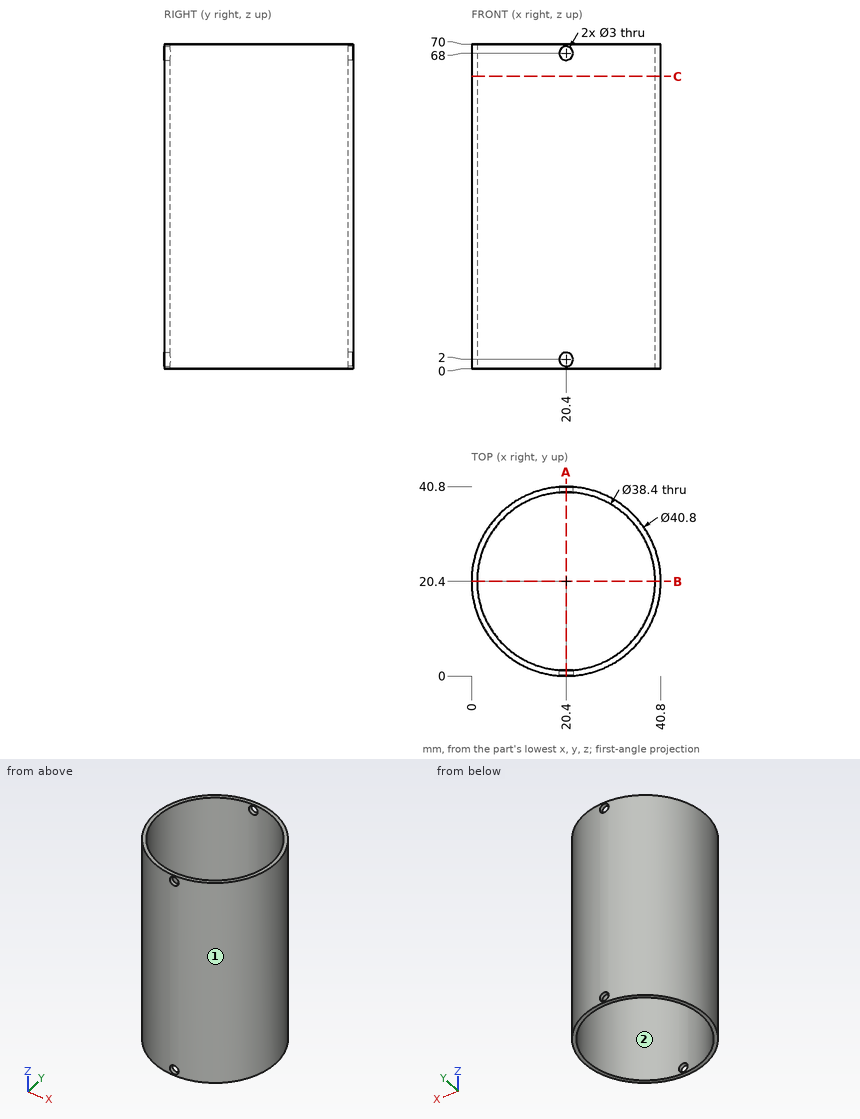
Design review of the part shown in the three views and the two pictorial views. Dimensions are in mm from the part's minimum x, y and z. Give positions to 0.01 mm unless a question says otherwise; leave off trailing zeros. Loops run counter-clockwise (first coordinate to the right, second up) from the corner with the lowest first, then second, coordinate; pieces in that order, holes last. Notation, with made-up numbers: (36.25, 88.25) -> (45.25, 88.25) arc R22 cw to (45.25, 108.25) -> close; hole circle Ø1 at (41.5, 32.5). An arc over 180 degrees is marked (long way). One line per item, written item: value.
Q1. We need section C-C on z = 63. Give the boundary of the cut face in (x, y).
Numbers:
outline: circle Ø40.8 at (20.4, 20.4); hole circle Ø38.4 at (20.4, 20.4)
Q2. We need section A-A on x = 20.4. Give the boundary of the cut face in (y, z), and give its area (3 significant figures).
Numbers:
outline: (0, 0) -> (1.2, 0) -> (1.2, 0.5) -> (0, 0.5) -> close; (0, 3.5) -> (1.2, 3.5) -> (1.2, 66.5) -> (0, 66.5) -> close; (0, 69.5) -> (1.2, 69.5) -> (1.2, 70) -> (0, 70) -> close; (39.6, 0) -> (40.8, 0) -> (40.8, 0.5) -> (39.6, 0.5) -> close; (39.6, 3.5) -> (40.8, 3.5) -> (40.8, 66.5) -> (39.6, 66.5) -> close; (39.6, 69.5) -> (40.8, 69.5) -> (40.8, 70) -> (39.6, 70) -> close
area: 154 mm^2
Q3. We need section B-B on y = 20.4. Give the boundary of the cut face in (x, z), and give its area (3 significant figures).
Numbers:
outline: (0, 0) -> (1.2, 0) -> (1.2, 70) -> (0, 70) -> close; (39.6, 0) -> (40.8, 0) -> (40.8, 70) -> (39.6, 70) -> close
area: 168 mm^2
Q4. For pin 1 Ø8 at (y, z) = (16.5, 61.5) entering from +X; pin 2 Ø1.5 at (x, z) = (32, 29) entering from +Y; pin 3 Ø1.5 at (x, z) = (22, 56) entering from +Y; pin 4 Ø12 at (y, z) = (5.5, 59) entering from -X, all flat-tipped, find the tip position at first contact; note any pin that passes through.
Numbers:
pin 1: stops at x = 40.8
pin 2: stops at y = 37.68
pin 3: stops at y = 40.78
pin 4: stops at x = 2.04
Q5. Draft analysis for pull direction Y (two halves, no side actions). For the marked faces 1 and 2, state which applies: pulls with the +Y half, pulls with the -Y half, needs draft (parallel to the pull), parting line crosses it, or undercut.
Numbers:
face 1: parting line crosses it
face 2: undercut
Q6. For L1, parallel to Z at x = 20.4, y = 40.25; L2, parallel to X at y = 20, z = 23; L3, parallel to Y at x = 24, z = 67.5, list the stretches that pass through material, from the lowest coordinate up.
Numbers:
L1: z = 0 to 0.5, 3.5 to 66.5, 69.5 to 70
L2: x = 0 to 1.2, 39.6 to 40.8
L3: y = 0.32 to 1.54, 39.26 to 40.48
